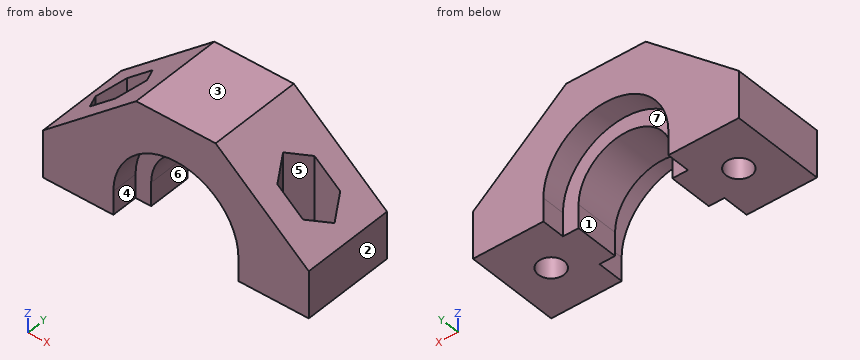
from build123d import *

# Parameters (mm, degrees)
EXTRUDE_1_DEPTH          = 3.4
EXTRUDE_2_DEPTH          = 5.6
EXTRUDE_3_DEPTH          = 3
SKETCH_5_R               = 1.65
CUT_EXTRUDE_2_DEPTH      = 4
CUT_EXTRUDE_2_DEPTH_BACK = 14
CUT_EXTRUDE_1_REACH      = 15


with BuildPart() as part:
    # 草图1 → 凸台-拉伸1 (new body)
    with BuildSketch(Plane(origin=(0, 0, 0), x_dir=(1, 0, 0), z_dir=(0, 1, 0))):
        with BuildLine():
            Line((-17, -3), (-5.082464074, -13))
            Line((-5.082464074, -13), (5.082464074, -13))
            Line((5.082464074, -13), (17, -3))
            Line((17, -3), (17, 0))
            Line((17, 0), (17, 3))
            Line((17, 3), (7.984491068, 3))
            Line((7.984491068, 3), (7.984491068, 0))
            Line((7.984491068, 0), (8, 0))
            ThreePointArc((8, 0), (0, -8), (-8, 0))
            Line((-8, 0), (-8, 3))
            Line((-8, 3), (-17, 3))
            Line((-17, 3), (-17, -3))
        make_face()
    extrude(amount=EXTRUDE_1_DEPTH)

    # 草图2 → 凸台-拉伸2 (add)
    with BuildSketch(Plane(origin=(0, 3.4, 0), x_dir=(1, 0, 0), z_dir=(0, 1, 0))):
        with BuildLine():
            Line((-17, -3), (-5.082464074, -13))
            Line((-5.082464074, -13), (5.082464074, -13))
            Line((5.082464074, -13), (17, -3))
            Line((17, -3), (17, 3))
            Line((17, 3), (6, 3))
            Line((6, 3), (6, 0))
            ThreePointArc((6, 0), (0, -6), (-6, 0))
            Line((-6, 0), (-6, 3))
            Line((-6, 3), (-17, 3))
            Line((-17, 3), (-17, -3))
        make_face()
    extrude(amount=EXTRUDE_2_DEPTH)

    # 草图3 → 凸台-拉伸3 (add)
    with BuildSketch(Plane(origin=(0, 9, 0), x_dir=(1, 0, 0), z_dir=(0, 1, 0))):
        with BuildLine():
            Line((-17, -3), (-5.082464074, -13))
            Line((-5.082464074, -13), (5.082464074, -13))
            Line((5.082464074, -13), (17, -3))
            Line((17, -3), (17, 3))
            Line((17, 3), (8, 3))
            Line((8, 3), (8, 0))
            ThreePointArc((8, 0), (0, -8), (-8, 0))
            Line((-8, 0), (-8, 3))
            Line((-8, 3), (-17, 3))
            Line((-17, 3), (-17, -3))
        make_face()
    extrude(amount=EXTRUDE_3_DEPTH)

    # 草图5 → 切除-拉伸2 (cut, two sides)
    with BuildSketch(Plane(origin=(0, 0, 0), x_dir=(-1, 0, 0), z_dir=(0, 0, -1))) as cut_extrude_2_sk:
        with Locations((12, 6)):
            Circle(SKETCH_5_R)
        with Locations((-12, 6)):
            Circle(SKETCH_5_R)
    extrude(amount=CUT_EXTRUDE_2_DEPTH, mode=Mode.SUBTRACT)
    extrude(cut_extrude_2_sk.sketch, amount=-CUT_EXTRUDE_2_DEPTH_BACK, mode=Mode.SUBTRACT)

    # 草图4 → 切除-拉伸1 (cut, up to next)
    with BuildSketch(Plane(origin=(0, 0, 0), x_dir=(-1, 0, 0), z_dir=(0, 0, -1)), mode=Mode.PRIVATE) as cut_extrude_1_sk1:
        Polygon((10.354551733, 3.15), (13.645448267, 3.15), (15.290896534, 6), (13.645448267, 8.85), (10.354551733, 8.85), (8.709103466, 6), align=None)
    cut_extrude_1_tool1 = extrude(cut_extrude_1_sk1.sketch, amount=-CUT_EXTRUDE_1_REACH, mode=Mode.PRIVATE) & part.part
    add(cut_extrude_1_tool1.solids().sort_by_distance((-12, 6, 0))[0], mode=Mode.SUBTRACT)
    # 草图4 → 切除-拉伸1 (cut, up to next)
    with BuildSketch(Plane(origin=(0, 0, 0), x_dir=(-1, 0, 0), z_dir=(0, 0, -1)), mode=Mode.PRIVATE) as cut_extrude_1_sk2:
        Polygon((-13.645448267, 3.15), (-10.354551733, 3.15), (-8.709103466, 6), (-10.354551733, 8.85), (-13.645448267, 8.85), (-15.290896534, 6), align=None)
    cut_extrude_1_tool2 = extrude(cut_extrude_1_sk2.sketch, amount=-CUT_EXTRUDE_1_REACH, mode=Mode.PRIVATE) & part.part
    add(cut_extrude_1_tool2.solids().sort_by_distance((12, 6, 0))[0], mode=Mode.SUBTRACT)


solid = part.part
For this review, take the finished solid that the model builds, in its own axes (mm). Face numbers are marked on the shaded views. A direction names the side the tool comes from. Round coordinates to 2 decimals unless told otherwise and drop trailing zeros. Write each loop counter-clockwise with the first axis right and the second up, starting at its lowest first coordinate (ties: lowest second). Pieces come first, ordered by that corner, then holes. Notation, with made-up numbers: (51, -23.75) -> (109, -23.75) arc R25 cw to (109, -2.75) -> close; hole circle Ø5 at (41.25, 44). An arc over 180 degrees is marked (long way). Put each result on its own line as item: value.
Q1. To check wall thickness, follow L1, parallel to X at y = 6, z = -1.75; L2, parallel to Y at x = 12, z = -2.35; L3, parallel to X at y = 1.75, z = -2.5. State the ranges of each line that lie inside material, in increasing order. Write a range as [from, to].
Determined:
L1: x = [-17, -13.65], [-10.35, -6], [6, 10.35], [13.65, 17]
L2: y = [0, 4.35], [7.65, 12]
L3: x = [-17, -8], [7.98, 17]
Q2. Machinability: for the marked faces 4, 5, 6 and 7, which of the approach directions +Z, -Z, +X, -X, +Y, -Y give a long, thin tool a straight path to every point of the face, cutting with its end or side? Answer none if there is none.
Determined:
face 4: -Z, -Y
face 5: +Z
face 6: -Z, +Y, -Y
face 7: -Z, +Y
Q3. Clearance check with flat-ended pins moving along their axes: pin 1 Ø5 at (x, y) = (-11.5, 10) entering from +Z; pin 2 Ø6.5 at (x, y) = (11, 7) entering from +Z; pin 3 Ø5.5 at (x, z) = (-4, 2.5) entering from +Y. State where each tip first meets the part, or that it passes through.
Determined:
pin 1: stops at z = 9.71
pin 2: stops at z = 10.76
pin 3: stops at y = 9
Q4. Consider section B-B on y = 5. State the section outline as (x, z) points, and give its area (3 significant figures).
Determined:
outline: (-17, -3) -> (-13.31, -3) -> (-13.31, 0) -> (-14.71, 0) -> (-14.71, 4.92) -> (-17, 3) -> close; (-10.69, -3) -> (-6, -3) -> (-6, 0) arc R6 cw to (6, 0) -> (6, -3) -> (10.69, -3) -> (10.69, 0) -> (9.29, 0) -> (9.29, 9.47) -> (5.08, 13) -> (-5.08, 13) -> (-9.29, 9.47) -> (-9.29, 0) -> (-10.69, 0) -> close; (13.31, -3) -> (17, -3) -> (17, 3) -> (14.71, 4.92) -> (14.71, 0) -> (13.31, 0) -> close
area: 238 mm^2
Q5. The part is to be moulded in two halves that separate along X. For the marked faces 1, 2 and 3, say which applies: released by +X, released by -X, zero draft, split by the parting line, or undercut.
Determined:
face 1: undercut
face 2: released by +X
face 3: zero draft
Q6. Consider section A-A on z = 0.75. State the section outline as (x, y) points.
Determined:
outline: (-17, 0) -> (-7.96, 0) -> (-7.96, 3.4) -> (-5.95, 3.4) -> (-5.95, 9) -> (-7.96, 9) -> (-7.96, 12) -> (-17, 12) -> close; (5.95, 3.4) -> (7.96, 3.4) -> (7.96, 0) -> (17, 0) -> (17, 12) -> (7.96, 12) -> (7.96, 9) -> (5.95, 9) -> close; hole (-15.29, 6) -> (-13.65, 3.15) -> (-10.35, 3.15) -> (-8.71, 6) -> (-10.35, 8.85) -> (-13.65, 8.85) -> close; hole (8.71, 6) -> (10.35, 3.15) -> (13.65, 3.15) -> (15.29, 6) -> (13.65, 8.85) -> (10.35, 8.85) -> close
Q7. Consider section D-D on z = 7. State the section outline as (x, y) points.
Determined:
outline: (-12.23, 0) -> (-3.87, 0) -> (-3.87, 3.4) -> (3.87, 3.4) -> (3.87, 0) -> (12.23, 0) -> (12.23, 3.15) -> (10.35, 3.15) -> (8.71, 6) -> (10.35, 8.85) -> (12.23, 8.85) -> (12.23, 12) -> (3.87, 12) -> (3.87, 9) -> (-3.87, 9) -> (-3.87, 12) -> (-12.23, 12) -> (-12.23, 8.85) -> (-10.35, 8.85) -> (-8.71, 6) -> (-10.35, 3.15) -> (-12.23, 3.15) -> close
Q8. Consider section C-C on x = 12. State the section outline as (y, z) points.
Determined:
outline: (0, -3) -> (4.35, -3) -> (4.35, 0) -> (3.15, 0) -> (3.15, 7.2) -> (0, 7.2) -> close; (7.65, -3) -> (12, -3) -> (12, 7.2) -> (8.85, 7.2) -> (8.85, 0) -> (7.65, 0) -> close
